Check sheet for the drawn part. Datum: minimum x, y, z corner. Units: mm. A direction names the side the tool comes from. Coordinates: 2 decimals unless noted, no trailing zeros. Order: outer loops, then holes, each group sorted by start corner. A loop starts at its lowest first (then second) coordinate and runs counter-clockwise, first axis right, second up. Notation, with made-up numbers: (76, -25.5) - (99, -25.5) arc R18 cw to (99, -12.5) - close; hole circle Ø6 at (-20, 73). An arc over 180 degrees is marked (long way). Return JSON: item names as keys, results as strings. Group by question number.
Item 1: Tool access check on the marked faces 1 and 2. Record the directions out of +Z, -Z, +X, -X, +Y, -Y that give a thin tool (end or side, any length) a straight path to the whole face; none if there is none.
Item 2: Section check D-D on y = 8.75. Enter the section's corners in (x, z), then the cut area to 3 significant figures.
Item 3: Scan lines: probe 1 along Y at (x, z) = (6.5, 8.75); probe 2 along Y at (x, z) = (6.5, 0.6); probe 3 along Z at (x, y) = (4.25, 8.5). Record each from-to range of solid material in increasing order.
Item 4: Section check C-C on z = 7.25. Enter the section's corners in (x, y), then the cut area to 3 significant figures.
Item 5: Draft check along X on the marked faces 3, 4 and 5. Enter one of: pulls with the +X half, pulls with the -X half, needs draft (parallel to the pull), parting line crosses it, or undercut.
Item 6: Gauge pin test, flat ends, axial feed: pin 1 (5 mm diameter, centred on y = 1.5, z = 9, fed in from -X); pin 2 (2 mm diameter, centred on x = 8.5, z = 7, fed in from -Y); pin 3 (1 mm diameter, centred on y = 5.5, z = 6, fed in from +X); pin 4 (3 mm diameter, centred on x = 6.5, y = 6.5, fed in from -Z) (1 decimal). Record the tip position at first contact, or that the pin passes through.
Item 7: Section check A-A on x = 6.5. Enter the section's corners in (y, z).
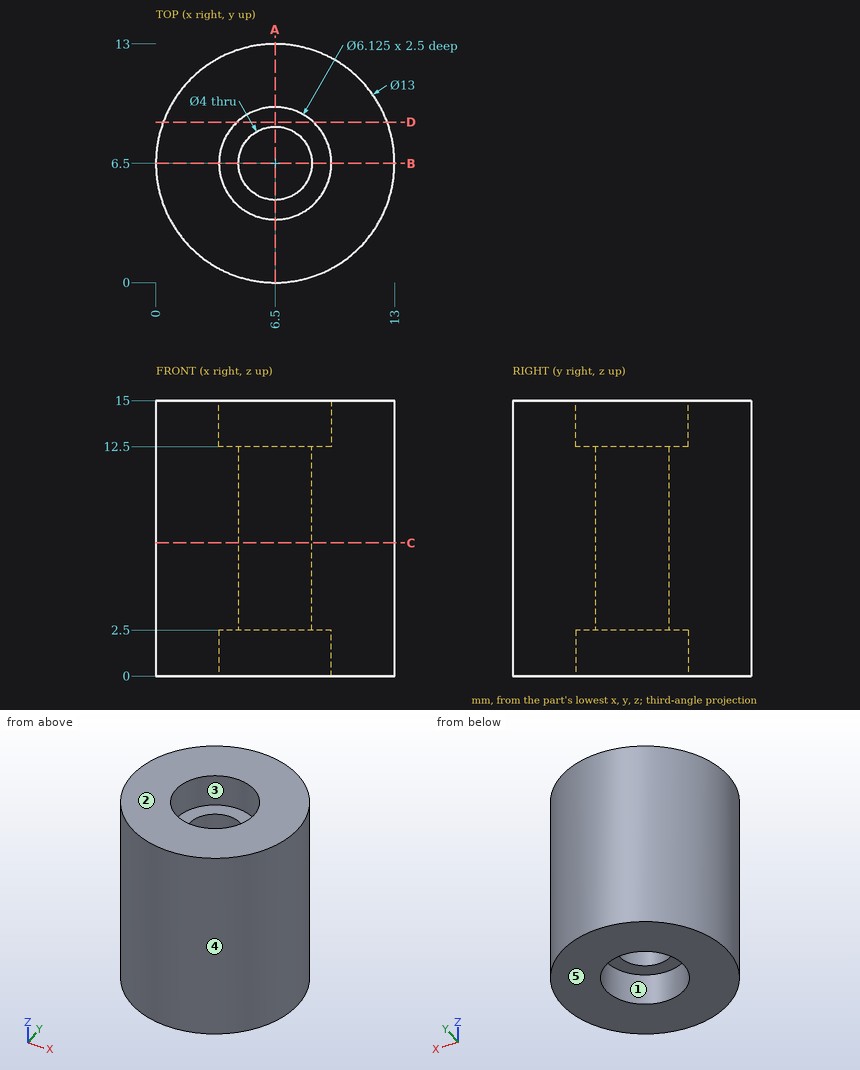
Computed:
{
 "1": {"face 1": "-Z", "face 2": "+Z, +X, -X, +Y, -Y"},
 "2": {"outline": "(0.4, 0) - (4.42, 0) - (4.42, 2.5) - (8.58, 2.5) - (8.58, 0) - (12.6, 0) - (12.6, 15) - (8.58, 15) - (8.58, 12.5) - (4.42, 12.5) - (4.42, 15) - (0.4, 15) - close", "area": "162 mm²"},
 "3": {"probe 1": "y = 0 to 4.5, 8.5 to 13", "probe 2": "y = 0 to 3.44, 9.56 to 13", "probe 3": "z = 2.5 to 12.5"},
 "4": {"outline": "circle Ø13 at (6.5, 6.5); hole circle Ø4 at (6.5, 6.5)", "area": "120 mm²"},
 "5": {"face 3": "undercut", "face 4": "parting line crosses it", "face 5": "needs draft"},
 "6": {"pin 1": "stops at x = 0.5", "pin 2": "stops at y = 0.08", "pin 3": "stops at x = 12.98", "pin 4": "passes through"},
 "7": {"outline": "(0, 0) - (3.44, 0) - (3.44, 2.5) - (4.5, 2.5) - (4.5, 12.5) - (3.44, 12.5) - (3.44, 15) - (0, 15) - close; (8.5, 2.5) - (9.56, 2.5) - (9.56, 0) - (13, 0) - (13, 15) - (9.56, 15) - (9.56, 12.5) - (8.5, 12.5) - close"}
}
